Source: CAD feature listing. Evaluate the final solid. Frame: model axes, mm. Face numbers are marked on the shaded views. A direction names the side the tool comes from. Give positions to 0.01 mm unless a question says otherwise; leave off trailing zeros. Loops run counter-clockwise (first coordinate to the right, second up) from the corner with the lowest first, then second, coordinate; pieces in that order, holes last. Notation, with made-up numbers: M 78.5,8 L 131.5,8 A17 cw 131.5,21 Z; hole C 89,2.5 d9. An arc over 180 degrees is marked long. Answer in a Markdown table with one row per item.
```python
from build123d import *

# Parameters (mm, degrees)
BOSS_EXTRUDE1_DEPTH = 70
FILLET1_R           = 2
FILLET2_R           = 2
FILLET3_R           = 1
FILLET4_R           = 1
FILLET5_R           = 1
FILLET6_R           = 1


with BuildPart() as part:
    # Sketch1 → Boss-Extrude1 (new body)
    with BuildSketch(Plane.XY):
        with BuildLine():
            Line((0, 35), (0, 0))
            Line((0, 0), (-5, 0))
            Line((-5, 0), (-5, 29.580398915))
            ThreePointArc((-5, 29.580398915), (-29.894915684, -2.508787808), (0, -30))
            Line((0, -30), (0, -32.5))
            ThreePointArc((0, -32.5), (5.527213221, -32.026550142), (10.893389008, -30.619994708))
            Line((10.893389008, -30.619994708), (9.114585792, -25.619994708))
            ThreePointArc((9.114585792, -25.619994708), (9.870035541, -23.320104454), (12.169925795, -24.075554203))
            Line((12.169925795, -24.075554203), (13.533846284, -26.773774571))
            Line((13.533846284, -26.773774571), (15.771374385, -31.245219635))
            ThreePointArc((15.771374385, -31.245219635), (-17.267698729, -30.443826642), (-34.910714286, -2.498405104))
            ThreePointArc((-34.910714286, -2.498405104), (-37.5, 0), (-34.910714286, 2.498405104))
            ThreePointArc((-34.910714286, 2.498405104), (-23.849065195, 25.616832148), (0, 35))
        make_face()
    extrude(amount=-BOSS_EXTRUDE1_DEPTH)

    # Fillet1
    fillet1_edges = [part.edges().sort_by_distance(p)[0] for p in [
        (-5, 0, -35),
    ]]
    fillet(fillet1_edges, radius=FILLET1_R)

    # Fillet2
    fillet2_edges = [part.edges().sort_by_distance(p)[0] for p in [
        (-5, 29.580398915, -35),
    ]]
    fillet(fillet2_edges, radius=FILLET2_R)

    # Fillet3
    fillet3_edges = [part.edges().sort_by_distance(p)[0] for p in [
        (0, -32.5, -35),
    ]]
    fillet(fillet3_edges, radius=FILLET3_R)

    # Fillet4
    fillet4_edges = [part.edges().sort_by_distance(p)[0] for p in [
        (15.771374385, -31.245219635, -35),
    ]]
    fillet(fillet4_edges, radius=FILLET4_R)

    # Fillet5
    fillet5_edges = [part.edges().sort_by_distance(p)[0] for p in [
        (-34.910714286, -2.498405104, -35),
        (-34.910714286, 2.498405104, -35),
    ]]
    fillet(fillet5_edges, radius=FILLET5_R)

    # Fillet6
    fillet6_edges = [part.edges().sort_by_distance(p)[0] for p in [
        (0, 35, -35),
    ]]
    fillet(fillet6_edges, radius=FILLET6_R)


solid = part.part
```
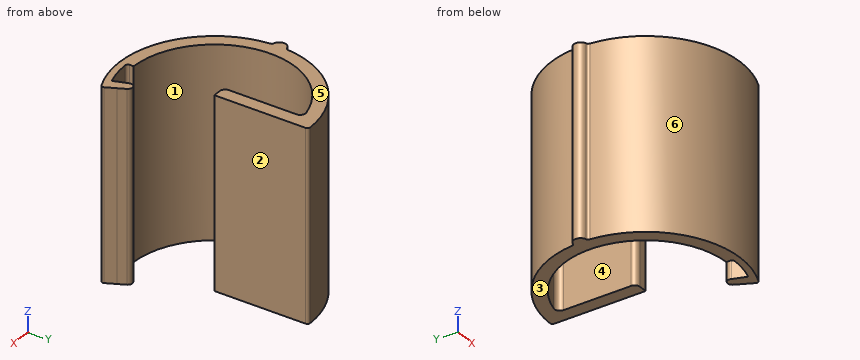
Q1. Section query D-D (x = 2). Output: boundary loops of the cut face in (y, z), plus the area to 3 significant figures.
Values follow:
| item | result |
|---|---|
| outline | M -34.94,-70 L -32.44,-70 L -32.44,0 L -34.94,0 Z |
| area | 175 mm^2 |
Q2. Ray query, probe 1 along Y at (x, z) = (-2, -63); probe 2 along X at (y, z) = (14, -45); probe 3 along Y at (x, z) = (-13, -36). Return the intervals inside material, ascending. Write a range as from..to.
Values follow:
| item | result |
|---|---|
| probe 1 | -34.94..-29.93, 0..34.94 |
| probe 2 | -32.08..-26.53, -5..0 |
| probe 3 | -32.5..-27.04, 27.04..32.5 |
Q3. Section query B-B (y = -15). Output: boundary loops of the cut face in (x, z), plus the area to 3 significant figures.
Values follow:
| item | result |
|---|---|
| outline | M -31.62,-70 L -25.98,-70 L -25.98,0 L -31.62,0 Z |
| area | 395 mm^2 |
Q4. Mould query, pull axis Y, two halves, no side actions, for the marked faces 4, 5 and 6. Classes: +Y half, -Y half, draft (parallel to the pull), parting line (faces both ways), or undercut.
Values follow:
| item | result |
|---|---|
| face 4 | undercut |
| face 5 | draft |
| face 6 | -Y half |
Q5. Reachability of the marked faces 1, 2 and 3 from +Z, -Z, +X, -X, +Y, -Y: full face, straight path, thin tool, end or side. Return the list, or none.
Values follow:
| item | result |
|---|---|
| face 1 | +Z, -Z |
| face 2 | +Z, -Z, +X, +Y |
| face 3 | -Z, +X, -X, +Y, -Y |
Q6. Contact query for flat-ended pins moving along their axis: pin 1 Ø6 at (y, z) = (20, -7.5) entering from +X; pin 2 Ø1.5 at (y, z) = (24.5, -41) entering from -X; pin 3 Ø1.5 at (y, z) = (6.5, -12) entering from -X; pin 4 Ø6 at (x, y) = (-1, -25) entering from +Z. Output: stop coordinate, or through.
Values follow:
| item | result |
|---|---|
| pin 1 | x = 0 |
| pin 2 | x = -25.71 |
| pin 3 | x = -34.52 |
| pin 4 | through |
Q7. Section query C-C (x = -26.5). Output: boundary loops of the cut face in (y, z), plus the area to 3 significant figures.
Values follow:
| item | result |
|---|---|
| outline | M -22.86,-70 L -14.06,-70 L -14.06,0 L -22.86,0 Z; M 14.06,-70 L 22.86,-70 L 22.86,0 L 14.06,0 Z |
| area | 1,230 mm^2 |
Q8. Section query A-A (x = -6). Output: boundary loops of the cut face in (y, z), plus the area to 3 significant figures.
Values follow:
| item | result |
|---|---|
| outline | M -34.48,-70 L -29.39,-70 L -29.39,0 L -34.48,0 Z; M 28.84,-70 L 34.48,-70 L 34.48,0 L 28.84,0 Z |
| area | 751 mm^2 |
